```python
from build123d import *

# Parameters (mm, degrees)
SKETCH_1_W           = 20
SKETCH_1_H           = 40
EXTRUDE_1_DEPTH      = 40
SKETCH_2_R           = 0.6
CUT_EXTRUDE_1_DEPTH  = 5
EXTRUDE_3_DEPTH      = 5
EXTRUDE_3_DEPTH_BACK = 45
SKETCH_3_R           = 3
SKETCH_4_R           = 1
CUT_EXTRUDE_2_DEPTH  = 5
FILLET_1_R           = 2


with BuildPart() as part:
    # ｽｹｯﾁ1 → ﾎﾞｽ - 押し出し1 (new body)
    with BuildSketch(Plane(origin=(0, 0, 0), x_dir=(0, 0, -1), z_dir=(1, 0, 0))):
        with Locations((18.409001804, -0.200935369)):
            Rectangle(SKETCH_1_W, SKETCH_1_H)
    extrude(amount=EXTRUDE_1_DEPTH)

    # ｽｹｯﾁ2 → ｶｯﾄ - 押し出し1 (cut)
    with BuildSketch(Plane(origin=(40, 0, 0), x_dir=(0, 0, -1), z_dir=(1, 0, 0))):
        with Locations((26.909001804, -18.700935369)):
            Circle(SKETCH_2_R)
        with Locations((26.909001804, -3.700935369)):
            Circle(SKETCH_2_R)
        with Locations(Location((9.909001804, -3.700935369, 0), (0, 0, 180))):
            Circle(SKETCH_2_R)
        with Locations(Location((9.909001804, -18.700935369, 0), (0, 0, 180))):
            Circle(SKETCH_2_R)
    extrude(amount=-CUT_EXTRUDE_1_DEPTH, mode=Mode.SUBTRACT)

    # ｽｹｯﾁ3 → ﾎﾞｽ - 押し出し3 (add, two sides: drawn at the far end of the back side and taken through both)
    with BuildSketch(Plane(origin=(40, 0, 0), x_dir=(0, 0, -1), z_dir=(1, 0, 0)).offset(-EXTRUDE_3_DEPTH_BACK)):
        with Locations((18.409001804, 11.299064631)):
            Circle(SKETCH_3_R)
    extrude(amount=EXTRUDE_3_DEPTH + EXTRUDE_3_DEPTH_BACK)

    # ｽｹｯﾁ4 → ｶｯﾄ - 押し出し2 (cut)
    with BuildSketch(Plane.ZY):
        with Locations((-11.409001804, -13.700935369)):
            Circle(SKETCH_4_R)
        with Locations((-25.409001804, -13.700935369)):
            Circle(SKETCH_4_R)
        with Locations(Location((-26.409001804, 2.299064631, 0), (0, 0, 180))):
            Circle(SKETCH_4_R)
        with Locations((-10.409001804, 2.299064631)):
            Circle(SKETCH_4_R)
        with Locations((-11.409001804, -10.700935369)):
            Circle(SKETCH_4_R)
        with Locations(Location((-25.409001804, -10.700935369, 0), (0, 0, 180))):
            Circle(SKETCH_4_R)
        with Locations((-18.409001804, -17.200935369)):
            Circle(SKETCH_4_R)
    extrude(amount=-CUT_EXTRUDE_2_DEPTH, mode=Mode.SUBTRACT)

    # ﾌｨﾚｯﾄ1
    fillet_1_edges = [part.edges().sort_by_distance(p)[0] for p in [
        (20, 19.799064631, -8.409001804),
        (20, 19.799064631, -28.409001804),
        (20, -20.200935369, -28.409001804),
        (20, -20.200935369, -8.409001804),
    ]]
    fillet(fillet_1_edges, radius=FILLET_1_R)


solid = part.part
```
Geometry check sheet. Reference: the model listing, model coordinates, mm. A direction names the side the tool comes from. Coordinates: 2 decimals unless noted, no trailing zeros. Write each loop counter-clockwise with the first axis right and the second up, starting at its lowest first coordinate (ties: lowest second). Pieces come first, ordered by that corner, then holes. Notation, with made-up numbers: (-6.5, 57.5) -> (-0.5, 57.5) arc R22 ccw to (-0.5, 90.5) -> close; hole circle Ø8 at (60.25, 45.25). An arc over 180 degrees is marked (long way). Use CSV: the item, a comma, the result in double quotes. Start each with the question number.
Item 1: Set-up check for faces 4 (the flat face through (5, 2, -10)), 5 (the flat face through (35, -4, -10)), 6 (the flat face through (-5, 11, -18)): record each of +Z, -Z, +X, -X, +Y, -Y from which the full face is reachable in a straight line by a thin tool's end or side.
Item 2: Cross-section at C-C, the plane y = 4. Record the cut outline in (x, z), plus the area to 3 significant figures.
Item 3: Mould release check, pull along Z, two halves, no side actions. Record for faces 1 (the flat face through (20, -20.201, -18)), 2 (the flat face through (35, -19, -27)), 3 (the cylindrical face through (20.28, -19.63, -27.81)): released by +Z, released by -Z, zero draft, split by the parting line, or undercut.
Item 4: Cross-section at D-D, the plane z = -22. Record the cut outline in (x, y).
Item 5: Thickness scan on line 1 (Z direction, x = 3.5, y = -11); line 2 (Z direction, x = 1, y = -10.5); line 3 (Y direction, x = 3, z = -25.5). Record the ranges inside material, lowest first.
Item 6: Cross-section at A-A, the plane x = 1. Record the cut outline in (y, z).
Item 7: Cross-section at B-B, the plane z = -16.75. Record the cut outline in (x, y), plus the area to 3 significant figures.
Item 8: Depth check by flat-ended pin: pin 1 Ø2.5 at (y, z) = (-10.7, -11.41) entering from +X; pin 2 Ø4 at (y, z) = (5, -24.5) entering from -X; pin 3 Ø1 at (y, z) = (-17.5, -18.5) entering from -X. Enter the tip coordinate at first touch or a pass-through.
Answers:
1,face 4,"-X"
1,face 5,"+X"
1,face 6,"+Z, -Z, -X, +Y, -Y"
2,outline,"(0, -28.41) -> (40, -28.41) -> (40, -8.41) -> (0, -8.41) -> close"
2,area,"800 mm^2"
3,face 1,"zero draft"
3,face 2,"undercut"
3,face 3,"released by -Z"
4,outline,"(0, -20.2) -> (40, -20.2) -> (40, 19.8) -> (0, 19.8) -> close"
5,line 1,"-28.41 to -26.36, -24.45 to -12.36, -10.45 to -8.41"
5,line 2,"-28.41 to -26.39, -24.43 to -12.39, -10.43 to -8.41"
5,line 3,"-20.2 to -14.7, -12.71 to -11.7, -9.71 to 1.88, 2.72 to 19.8"
6,outline,"(-20.2, -26.41) arc R2 ccw to (-18.2, -28.41) -> (17.8, -28.41) arc R2 ccw to (19.8, -26.41) -> (19.8, -10.41) arc R2 ccw to (17.8, -8.41) -> (-18.2, -8.41) arc R2 ccw to (-20.2, -10.41) -> close; hole circle Ø2 at (-17.2, -18.41); hole circle Ø2 at (-13.7, -25.41); hole circle Ø2 at (-13.7, -11.41); hole circle Ø2 at (-10.7, -25.41); hole circle Ø2 at (-10.7, -11.41); hole circle Ø2 at (2.3, -26.41); hole circle Ø2 at (2.3, -10.41)"
7,outline,"(-5, 8.8) -> (0, 8.8) -> (0, -20.2) -> (40, -20.2) -> (40, 8.8) -> (45, 8.8) -> (45, 13.8) -> (40, 13.8) -> (40, 19.8) -> (0, 19.8) -> (0, 13.8) -> (-5, 13.8) -> close"
7,area,"1,650 mm^2"
8,pin 1,"x = 40"
8,pin 2,"x = 0"
8,pin 3,"x = 5"
